```python
from build123d import *

# Parameters (mm, degrees)
BOSS_EXTRUDE2_DEPTH      = 12
BOSS_EXTRUDE2_DEPTH_BACK = 3
BOSS_EXTRUDE3_DEPTH      = 3
SKETCH6_W                = 5
SKETCH6_H                = 2.1
CUT_EXTRUDE1_DEPTH       = 10
SKETCH7_W                = 4.2
SKETCH7_H                = 4.5
CUT_EXTRUDE2_DEPTH       = 10
FILLET1_R                = 1
SKETCH8_W                = 4
SKETCH8_H                = 4
BOSS_EXTRUDE4_DEPTH      = 15
FILLET2_R                = 1.2
SKETCH9_R                = 0.75
CUT_EXTRUDE3_DEPTH       = 83.553600769
SKETCH10_R               = 3.5
CUT_EXTRUDE4_DEPTH       = 1.5
FILLET3_R                = 0.3


with BuildPart() as part:
    # Sketch3 → Boss-Extrude2 (new, two sides: drawn at the far end of the back side and taken through both)
    with BuildSketch(Plane.XY.offset(-BOSS_EXTRUDE2_DEPTH_BACK)):
        with BuildLine():
            Line((-69.81, 19.47), (-34.625063383, 19.47))
            ThreePointArc((-34.625063383, 19.47), (-32.763487521, 19.110531791), (-31.169582594, 18.083814123))
            Line((-31.169582594, 18.083814123), (-26.833005647, 13.937237175))
            ThreePointArc((-26.833005647, 13.937237175), (-26.514224661, 13.731893642), (-26.141909489, 13.66))
            Line((-26.141909489, 13.66), (-1.5, 13.66))
            ThreePointArc((-1.5, 13.66), (2.035533906, 12.195533906), (3.5, 8.66))
            Line((3.5, 8.66), (3.5, 1.5))
            ThreePointArc((3.5, 1.5), (2.035533906, -2.035533906), (-1.5, -3.5))
            Line((-1.5, -3.5), (-26.141909489, -3.5))
            ThreePointArc((-26.141909489, -3.5), (-26.514224661, -3.571893642), (-26.833005647, -3.777237175))
            Line((-26.833005647, -3.777237175), (-31.169582594, -7.923814123))
            ThreePointArc((-31.169582594, -7.923814123), (-32.763487521, -8.950531791), (-34.625063383, -9.31))
            Line((-34.625063383, -9.31), (-69.81, -9.31))
            ThreePointArc((-69.81, -9.31), (-73.345533906, -7.845533906), (-74.81, -4.31))
            Line((-74.81, -4.31), (-74.81, 14.47))
            ThreePointArc((-74.81, 14.47), (-73.345533906, 18.005533906), (-69.81, 19.47))
        make_face()
        with BuildLine():
            Line((-69.81, 17.47), (-34.625063383, 17.47))
            ThreePointArc((-34.625063383, 17.47), (-33.508117866, 17.254319075), (-32.55177491, 16.638288474))
            Line((-32.55177491, 16.638288474), (-28.215197962, 12.491711526))
            ThreePointArc((-28.215197962, 12.491711526), (-27.258855006, 11.875680925), (-26.141909489, 11.66))
            Line((-26.141909489, 11.66), (-1.5, 11.66))
            ThreePointArc((-1.5, 11.66), (0.621320344, 10.781320344), (1.5, 8.66))
            Line((1.5, 8.66), (1.5, 1.5))
            ThreePointArc((1.5, 1.5), (0.621320344, -0.621320344), (-1.5, -1.5))
            Line((-1.5, -1.5), (-26.141909489, -1.5))
            ThreePointArc((-26.141909489, -1.5), (-27.258855006, -1.715680925), (-28.215197962, -2.331711526))
            Line((-28.215197962, -2.331711526), (-32.55177491, -6.478288474))
            ThreePointArc((-32.55177491, -6.478288474), (-33.508117866, -7.094319075), (-34.625063383, -7.31))
            Line((-34.625063383, -7.31), (-69.81, -7.31))
            ThreePointArc((-69.81, -7.31), (-71.931320344, -6.431320344), (-72.81, -4.31))
            Line((-72.81, -4.31), (-72.81, 14.47))
            ThreePointArc((-72.81, 14.47), (-71.931320344, 16.591320344), (-69.81, 17.47))
        make_face(mode=Mode.SUBTRACT)
    extrude(amount=BOSS_EXTRUDE2_DEPTH + BOSS_EXTRUDE2_DEPTH_BACK)

    # Sketch5 → Boss-Extrude3 (add)
    with BuildSketch(Plane(origin=(0, 0, -3), x_dir=(-1, 0, 0), z_dir=(0, 0, -1))):
        with BuildLine():
            Line((72.81, 14.47), (72.81, -4.31))
            ThreePointArc((72.81, -4.31), (71.931320344, -6.431320344), (69.81, -7.31))
            Line((69.81, -7.31), (34.625063383, -7.31))
            ThreePointArc((34.625063383, -7.31), (33.508117866, -7.094319075), (32.55177491, -6.478288474))
            Line((32.55177491, -6.478288474), (28.215197962, -2.331711526))
            ThreePointArc((28.215197962, -2.331711526), (27.258855006, -1.715680925), (26.141909489, -1.5))
            Line((26.141909489, -1.5), (1.5, -1.5))
            ThreePointArc((1.5, -1.5), (-0.621320344, -0.621320344), (-1.5, 1.5))
            Line((-1.5, 1.5), (-1.5, 8.66))
            ThreePointArc((-1.5, 8.66), (-0.621320344, 10.781320344), (1.5, 11.66))
            Line((1.5, 11.66), (26.141909489, 11.66))
            ThreePointArc((26.141909489, 11.66), (27.258855006, 11.875680925), (28.215197962, 12.491711526))
            Line((28.215197962, 12.491711526), (32.55177491, 16.638288474))
            ThreePointArc((32.55177491, 16.638288474), (33.508117866, 17.254319075), (34.625063383, 17.47))
            Line((34.625063383, 17.47), (69.81, 17.47))
            ThreePointArc((69.81, 17.47), (71.931320344, 16.591320344), (72.81, 14.47))
        make_face()
    extrude(amount=-BOSS_EXTRUDE3_DEPTH)

    # Sketch6 → Cut-Extrude1 (cut)
    with BuildSketch(Plane.ZY.offset(74.81)):
        with Locations((9.5, 6.13)):
            Rectangle(SKETCH6_W, SKETCH6_H)
        with Locations((9.5, 4.03)):
            Rectangle(SKETCH6_W, SKETCH6_H)
    extrude(amount=-CUT_EXTRUDE1_DEPTH, mode=Mode.SUBTRACT)

    # Sketch7 → Cut-Extrude2 (cut)
    with BuildSketch(Plane(origin=(0, 13.66, 0), x_dir=(1, 0, 0), z_dir=(0, 1, 0))):
        with Locations((-6.6, -9.75)):
            Rectangle(SKETCH7_W, SKETCH7_H)
    extrude(amount=-CUT_EXTRUDE2_DEPTH, mode=Mode.SUBTRACT)

    # Fillet1
    fillet1_edges = [part.edges().sort_by_distance(p)[0] for p in [
        (-73.81, 2.98, 12),
        (-73.81, 7.18, 12),
        (-72.81, 5.08, 7),
        (-73.81, 2.98, 7),
        (-73.81, 7.18, 7),
        (-74.81, 7.18, 9.5),
        (-72.81, 2.98, 9.5),
        (-72.81, 7.18, 9.5),
        (-74.81, 5.08, 7),
        (-74.81, 2.98, 9.5),
        (-4.5, 12.66, 12),
        (-8.7, 11.66, 9.75),
        (-8.7, 12.66, 12),
        (-6.6, 11.66, 7.5),
        (-8.7, 12.66, 7.5),
        (-4.5, 11.66, 9.75),
        (-4.5, 12.66, 7.5),
        (-4.5, 13.66, 9.75),
        (-6.6, 13.66, 7.5),
        (-8.7, 13.66, 9.75),
    ]]
    fillet(fillet1_edges, radius=FILLET1_R - 0.0001)  # a hair under: the kernel refuses the full size

    # Sketch8 → Boss-Extrude4 (add, through all)
    with BuildSketch(Plane.XY.offset(12)):
        with Locations((-76.81, 12.47)):
            Rectangle(SKETCH8_W, SKETCH8_H)
        with Locations((-3.5, -5.5)):
            Rectangle(SKETCH8_W, SKETCH8_H)
    extrude(amount=-BOSS_EXTRUDE4_DEPTH)

    # Fillet2
    fillet2_edges = [part.edges().sort_by_distance(p)[0] for p in [
        (-1.5, -3.5, 4.5),
        (-74.81, 14.47, 4.5),
        (-74.81, 10.47, 4.5),
        (-78.81, 10.47, 4.5),
        (-78.81, 14.47, 4.5),
        (-1.5, -7.5, 4.5),
        (-5.5, -7.5, 4.5),
        (-5.5, -3.5, 4.5),
    ]]
    fillet(fillet2_edges, radius=FILLET2_R)

    # Sketch9 → Cut-Extrude3 (cut, through all)
    with BuildSketch(Plane.XY.offset(12)):
        with Locations((-76.81, 12.47)):
            Circle(SKETCH9_R)
        with Locations((-3.5, -5.5)):
            Circle(SKETCH9_R)
    extrude(amount=-CUT_EXTRUDE3_DEPTH, mode=Mode.SUBTRACT)

    # Sketch10 → Cut-Extrude4 (cut)
    with BuildSketch(Plane(origin=(0, 0, -3), x_dir=(-1, 0, 0), z_dir=(0, 0, -1))):
        with Locations((62.81, 5.08)):
            Circle(SKETCH10_R)
    extrude(amount=-CUT_EXTRUDE4_DEPTH, mode=Mode.SUBTRACT)

    # Fillet3
    fillet3_edges = [part.edges().sort_by_distance(p)[0] for p in [
        (-59.31, 5.08, -3),
    ]]
    fillet(fillet3_edges, radius=FILLET3_R)


solid = part.part
```
Geometry check sheet. Reference: the model listing, model coordinates, mm. A direction names the side the tool comes from. Round coordinates to 2 decimals unless told otherwise and drop trailing zeros. Order: outer loops, then holes, each group sorted by start corner. A loop starts at its lowest first (then second) coordinate and runs counter-clockwise, first axis right, second up. Notation, with made-up numbers: (52.5, 48.5) - (85.5, 48.5) arc R26 ccw to (85.5, 80.5) - close; hole circle Ø8 at (56, -29.75). An arc over 180 degrees is marked (long way). Use a Markdown table: item, result. Add a question column.
1) Mould release check, pull along Y, two halves, no side actions. Record for faces 6 (the cylindrical face through (0.6, 10.8, 5.9)), 7 (the cylindrical face through (-32.74, -8.94, 4.39)), 8 (the flat face through (-14, 13.66, 4)), 9 (the flat face through (1.5, 5, 6)): released by +Y, released by -Y, zero draft, split by the parting line, or undercut.
2) Section check D-D (z = 5). Count the separate pieces of the cut face and the enclosed holes in it, then the cut area to 3 significant figures.
3) Section check A-A (x = -76.81). Record the cut outline in (y, z).
4) Thickness scan on line 1 along Y through (x, z) = (-3.5, 2); line 2 along Y through (x, z) = (-49, 11); line 3 along Y through (x, z) = (-76.81, 1.5). Record the ranges inside material, lowest first.
5) Section check C-C (x = -62.81). Record the cut outline in (y, z).
6) Gauge pin test, flat ends, axial feed: P1, Ø9, axis at x = -62.81, y = 5.08, coming from the -Z side; P2, Ø1.3, axis at x = -77, z = 5.5, coming from the -Y side; P3, Ø0.9, axis at x = -76.81, y = 12.47, coming from the +Z side; P4, Ø7.5, axis at x = -17, z = 2, coming from the -Y side. Record the tip position at first contact, or that the pin passes through.
7) Set-up check for faces 1 (the flat face through (-52, -7.31, 6)), 2 (the flat face through (-1.5, -5, 5)), 3 (the flat face through (-28.97, -5.82, 4.39)), 4 (the flat face through (-77, 14.47, 5)), 5 (the flat face through (-77, 10.47, 5)): record each of +Z, -Z, +X, -X, +Y, -Y from which the full face is reachable in a straight line by a thin tool's end or side.
Established:
| question | item | result |
|---|---|---|
| 1 | face 6 | undercut |
| 1 | face 7 | released by -Y |
| 1 | face 8 | released by +Y |
| 1 | face 9 | undercut |
| 2 | separate pieces | 1 |
| 2 | enclosed holes | 3 |
| 2 | area | 412 mm2 |
| 3 | outline | (10.47, -3) - (11.72, -3) - (11.72, 12) - (10.47, 12) - close; (13.22, -3) - (14.47, -3) - (14.47, 12) - (13.22, 12) - close |
| 4 | line 1 | -7.5 to -6.25, -4.75 to -1.5, 11.66 to 13.66 |
| 4 | line 2 | -9.31 to -7.31, 17.47 to 19.47 |
| 4 | line 3 | 10.47 to 11.72, 13.22 to 14.47 |
| 5 | outline | (-9.31, -3) - (1.28, -3) arc R0.3 ccw to (1.58, -2.7) - (1.58, -1.5) - (8.58, -1.5) - (8.58, -2.7) arc R0.3 ccw to (8.88, -3) - (19.47, -3) - (19.47, 12) - (17.47, 12) - (17.47, 0) - (-7.31, 0) - (-7.31, 12) - (-9.31, 12) - close |
| 6 | P1 | z = -3 |
| 6 | P2 | y = 10.47 |
| 6 | P3 | through |
| 6 | P4 | y = -3.5 |
| 7 | face 1 | +Z |
| 7 | face 2 | +Z, -Z, +X, -Y |
| 7 | face 3 | +Z, -Z, -Y |
| 7 | face 4 | +Z, -Z, -X, +Y |
| 7 | face 5 | +Z, -Z, -X, -Y |
